Part print with two shaded views. Sizes in mm from the minimum x, y, z corner. Round coordinates to 2 decimals unless told otherwise and drop trailing zeros. Write each loop counter-clockwise with the first axis right and the second up, starting at its lowest first coordinate (ties: lowest second). Pieces come first, ordered by that corner, then holes.
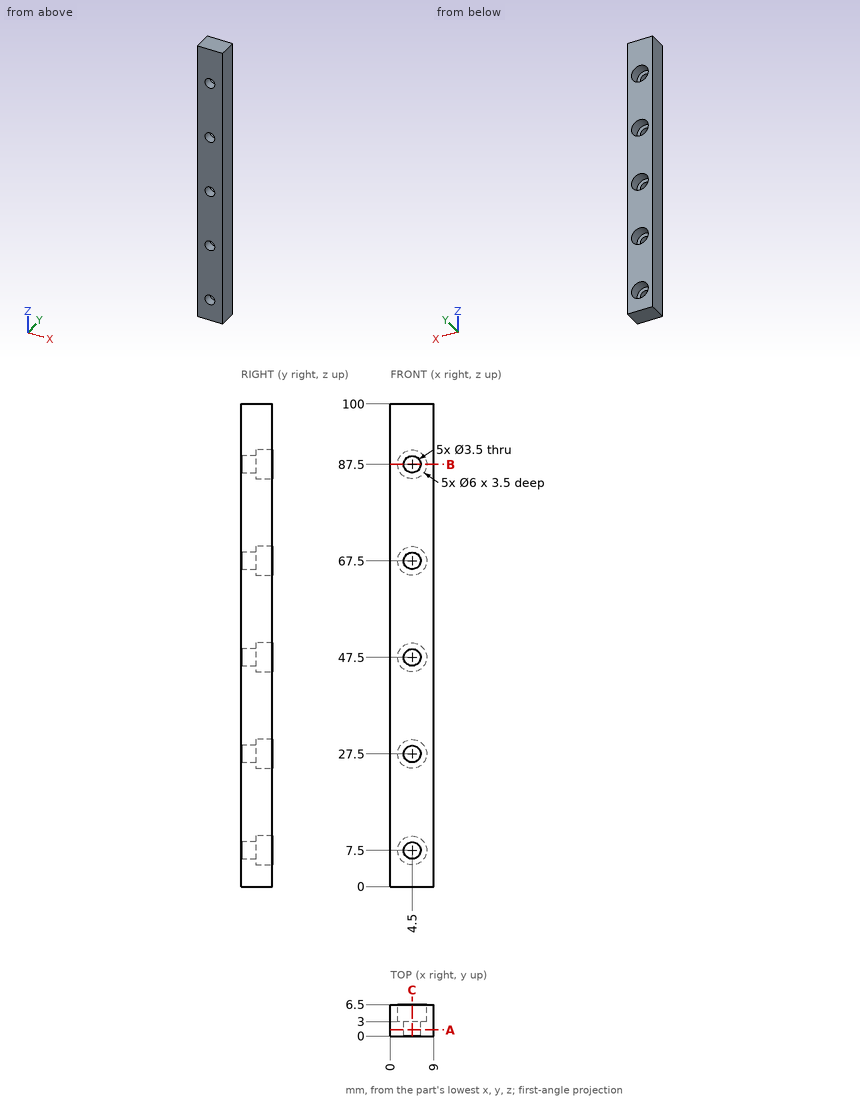
Q1. Cut at C-C on x = 4.5. State how many separate pieces and enclosed holes the cut face has, plus the area to 4 significant figures.
Values follow:
separate pieces: 6
enclosed holes: 0
area: 492.5 mm2
Q2. Drop a flat-ended pin along its axis: pin 1 (3 mm diameter, centred on x = 5, z = 47.5, fed in from +Y). Give the stop position or say it passes through.
Values follow:
pin 1: stops at y = 3
Q3. Wall check: L1, parallel to X at y = 5.4, z = 27.5; L2, parallel to Z at x = 5.25, y = 2.5; L3, parallel to Z at x = 5.75, y = 2.5. Give the ranges that are in metal, low to high.
Values follow:
L1: x = 0 to 1.5, 7.5 to 9
L2: z = 0 to 5.92, 9.08 to 25.92, 29.08 to 45.92, 49.08 to 65.92, 69.08 to 85.92, 89.08 to 100
L3: z = 0 to 6.28, 8.72 to 26.28, 28.72 to 46.28, 48.72 to 66.28, 68.72 to 86.28, 88.72 to 100
Q4. Cut at B-B on z = 87.5. Write the cut outline in (x, y), plus the area to 3 significant figures.
Values follow:
outline: (0, 0) - (2.75, 0) - (2.75, 3) - (1.5, 3) - (1.5, 6.5) - (0, 6.5) - close; (6.25, 0) - (9, 0) - (9, 6.5) - (7.5, 6.5) - (7.5, 3) - (6.25, 3) - close
area: 27.0 mm2
Q5. Cut at A-A on y = 1.25. Write the cut outline in (x, z).
Values follow:
outline: (0, 0) - (9, 0) - (9, 100) - (0, 100) - close; hole circle Ø3.5 at (4.5, 7.5); hole circle Ø3.5 at (4.5, 27.5); hole circle Ø3.5 at (4.5, 47.5); hole circle Ø3.5 at (4.5, 67.5); hole circle Ø3.5 at (4.5, 87.5)
